Input: dimensioned drawing with shaded views. Units: mm. Origin: part minimum x, y, z. Give positions to 0.01 mm unless a question says otherwise; leave off trailing zeros. Loops run counter-clockwise (first coordinate to the right, second up) from the corner with the lowest first, then second, coordinate; pieces in that order, holes last. Notation, with made-up numbers: M 42.25,-7 L 56.25,-7 A13 cw 56.25,-2 Z; hole C 81,18 d4. An arc over 180 degrees is marked long. Answer in a Markdown table with one row per item.
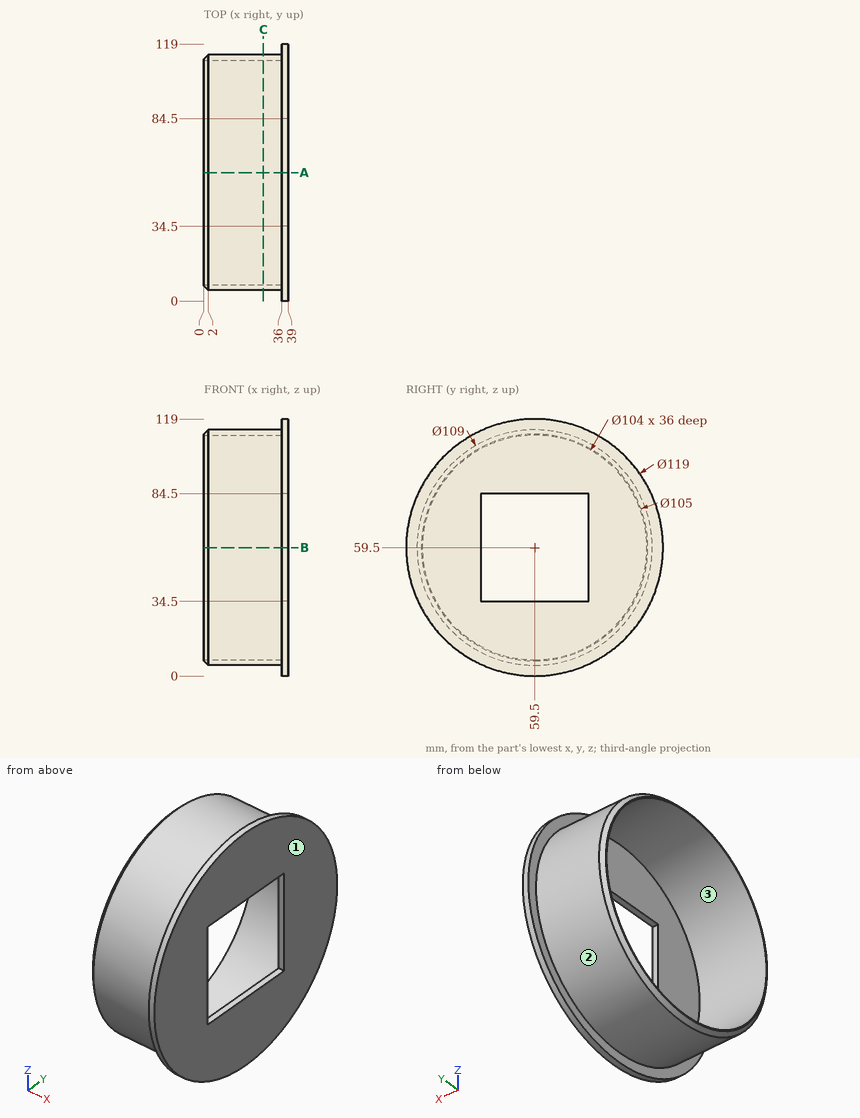
Q1. Contact query for flat-ended pins moving along their axis: pin 1 Ø2 at (x, y) = (21, 81) entering from -Z; pin 2 Ø3.5 at (x, z) = (37.5, 51.5) entering from -Y; pin 3 Ø4 at (x, z) = (14.5, 84.5) entering from -Y. Output: stop coordinate, or through.
Values follow:
| item | result |
|---|---|
| pin 1 | z = 9 |
| pin 2 | y = 0.33 |
| pin 3 | y = 10.09 |
Q2. Ray query, probe 1 along Y at (x, z) = (9, 59); probe 2 along Z at (x, y) = (6.5, 29). Return the intervals inside material, ascending. Write a range as from..to.
Values follow:
| item | result |
|---|---|
| probe 1 | 5..7.5, 111.5..114 |
| probe 2 | 14.33..17.38, 101.62..104.67 |
Q3. Mould query, pull axis Z, two halves, no side actions, for the marked faces 1, 2 and 3. Classes: +Z half, -Z half, draft (parallel to the pull), parting line (faces both ways), or undercut.
Values follow:
| item | result |
|---|---|
| face 1 | draft |
| face 2 | parting line |
| face 3 | undercut |
Q4. Section query A-A (y = 59.5). Output: boundary loops of the cut face in (x, z), plus the area to 3 significant figures.
Values follow:
| item | result |
|---|---|
| outline | M 0,7 L 2,5 L 36,5 L 36,0 L 39,0 L 39,34.5 L 36,34.5 L 36,7.5 L 0,7.5 Z; M 0,111.5 L 36,111.5 L 36,84.5 L 39,84.5 L 39,119 L 36,119 L 36,114 L 2,114 L 0,112 Z |
| area | 383 mm^2 |
Q5. Section query C-C (x = 27.5). Output: boundary loops of the cut face in (y, z), plus the area to 3 significant figures.
Values follow:
| item | result |
|---|---|
| outline | C 59.5,59.5 d109; hole C 59.5,59.5 d104 |
| area | 836 mm^2 |
